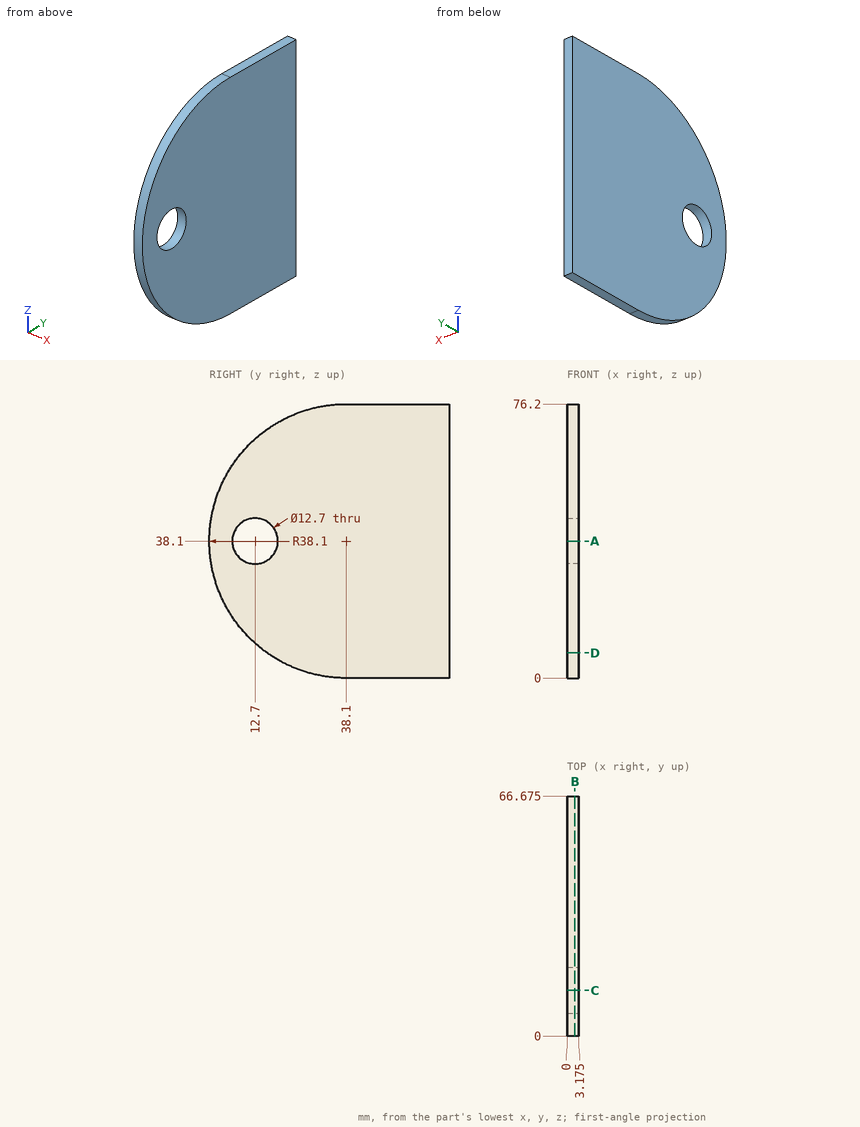
Verification items for this drawing (mm, ordinates from the low corner). Coordinates: 2 decimals unless noted, no trailing zeros. Loops run counter-clockwise (first coordinate to the right, second up) from the corner with the lowest first, then second, coordinate; pieces in that order, holes last. Notation, with made-up numbers: (-20, -24) -> (29, -24) arc R18 ccw to (29, 2) -> close; hole circle Ø1 at (35, 38). An arc over 180 degrees is marked (long way). Put each result on its own line as item: value.
1. Section check D-D, the plane z = 7. Record the boundary of the cut face in (x, y) (3 decimals), then the cut area to 3 significant figures.
Result set:
outline: (0, 16.091) -> (3.175, 16.091) -> (3.175, 66.675) -> (0, 66.675) -> close
area: 161 mm^2
2. Section check C-C, the plane y = 12.7. Record the boundary of the cut face in (x, z) (3 decimals).
Result set:
outline: (0, 9.702) -> (3.175, 9.702) -> (3.175, 31.75) -> (0, 31.75) -> close; (0, 44.45) -> (3.175, 44.45) -> (3.175, 66.498) -> (0, 66.498) -> close
3. Section check A-A, the plane z = 38.1. Record the boundary of the cut face in (x, y) (3 decimals), then the cut area to 3 significant figures.
Result set:
outline: (0, 0) -> (3.175, 0) -> (3.175, 6.35) -> (0, 6.35) -> close; (0, 19.05) -> (3.175, 19.05) -> (3.175, 66.675) -> (0, 66.675) -> close
area: 171 mm^2
4. Gauge pin test, flat ends, axial feed: P1, Ø1, axis at x = 3, z = 49, coming from the -Y side; P2, Ø1.5, axis at x = 3, z = 56.5, coming from the -Y side. Record the tip position at first contact, or that the pin passes through.
Result set:
P1: stops at y = 1.45
P2: stops at y = 4.33
5. Section check B-B, the plane x = 2.1. Record the boundary of the cut face in (y, z) (3 decimals), then the cut area to 3 significant figures.
Result set:
outline: (38.1, 0) -> (66.675, 0) -> (66.675, 76.2) -> (38.1, 76.2) arc R38.1 ccw to start; hole circle Ø12.7 at (12.7, 38.1)
area: 4,330 mm^2
6. Thickness scan on line 1 (Y direction, x = 1.1, z = 38.1) (3 decimals); line 2 (Z direction, x = 2.7, y = 14); line 3 (Z direction, x = 1.25, y = 16). Record the ranges inside material, lowest first.
Result set:
line 1: y = 0 to 6.35, 19.05 to 66.675
line 2: z = 8.59 to 31.88, 44.32 to 67.61
line 3: z = 7.06 to 32.67, 43.53 to 69.14
